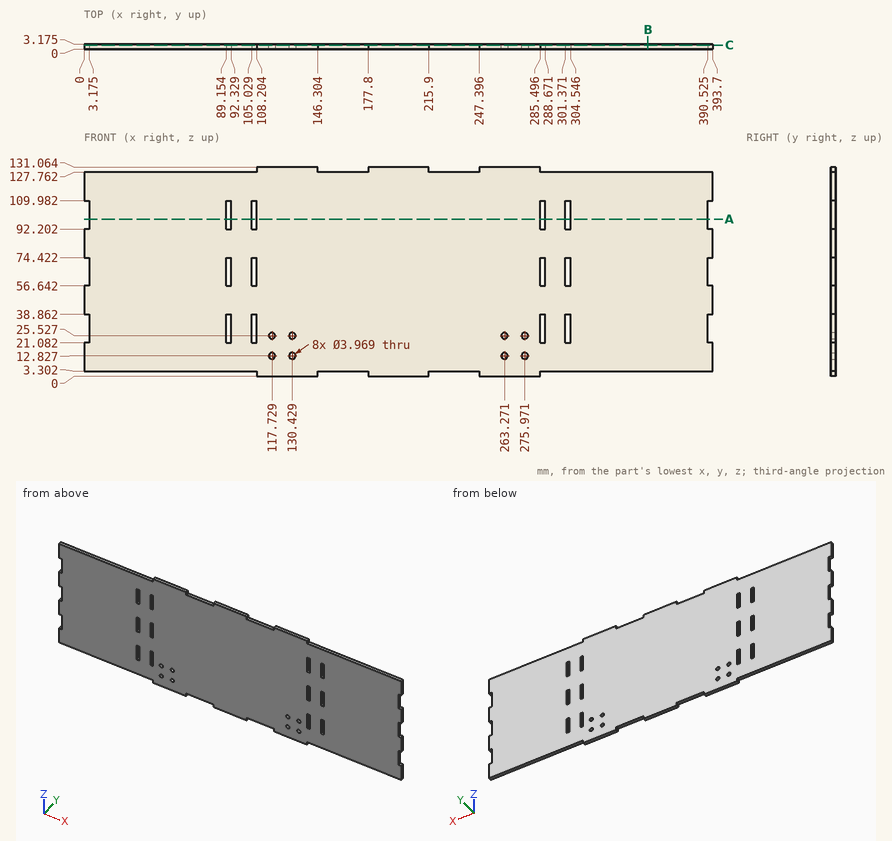
Answer from the drawing. Dimensions are ordinates in mm from the lowest x, y and z of the part. Round coordinates to 2 decimals unless told otherwise and drop trailing zeros. Loops run counter-clockwise (first coordinate to the right, second up) from the corner with the lowest first, then second, coordinate; pieces in that order, holes last. Notation, with made-up numbers: (30, 62.25) - (83, 62.25) arc R33 cw to (83, 97.25) - close; hole circle Ø8 at (75.5, 54.25). An arc over 180 degrees is marked (long way). Return JSON: item names as keys, results as strings. Group by question number.
1. Each of these flat-tipped pins is pushed along its axis until it touches: P1, Ø1.6, axis at y = 2, z = 64.5, coming from the +X side (3 decimals); P2, Ø2.5, axis at x = 117.729, z = 25.527, coming from the +Y side; P3, Ø1.6, axis at x = 392, y = 1.5, coming from the -Z side; P4, Ø1, axis at y = 1.5, z = 129.5, coming from the +X side. Where does it stop, or does it pass through?
2. The part is cut by section B-B on x = 353. Determine the outline of the cut face in (y, z) (1 decimal), then the cut area to 3 significant figures.
3. Consider probe 1 along X at (y, z) = (2.35, 68) (1 decimal); probe 2 along X at (y, z) = (1.9, 14); probe 3 along Z at (x, y) = (53.5, 1.7). Determine where each line is inside the solid, lowest interval first.
4. The part is cut by section C-C on y = 2.4. State how many separate pieces and enclosed holes the cut face has, then the cut area to 3 significant figures.
5. The part is cut by section A-A on z = 98.5. Determine the outline of the cut face in (x, y) (1 decimal), then the cut area to 3 significant figures.
Resolved:
{
 "1": {"P1": "stops at x = 390.525", "P2": "passes through", "P3": "stops at z = 3.3", "P4": "stops at x = 285.5"},
 "2": {"outline": "(0, 3.3) - (3.2, 3.3) - (3.2, 127.8) - (0, 127.8) - close", "area": "395 mm²"},
 "3": {"probe 1": "x = 3.2 to 89.2, 92.3 to 105, 108.2 to 285.5, 288.7 to 301.4, 304.5 to 390.5", "probe 2": "x = 0 to 116.13, 119.33 to 128.83, 132.03 to 261.67, 264.87 to 274.37, 277.57 to 393.7", "probe 3": "z = 3.3 to 127.76"},
 "4": {"separate pieces": "1", "enclosed holes": "20", "area": "48,600 mm²"},
 "5": {"outline": "(3.2, 0) - (89.2, 0) - (89.2, 3.2) - (3.2, 3.2) - close; (92.3, 0) - (105, 0) - (105, 3.2) - (92.3, 3.2) - close; (108.2, 0) - (285.5, 0) - (285.5, 3.2) - (108.2, 3.2) - close; (288.7, 0) - (301.4, 0) - (301.4, 3.2) - (288.7, 3.2) - close; (304.5, 0) - (390.5, 0) - (390.5, 3.2) - (304.5, 3.2) - close", "area": "1,190 mm²"}
}
